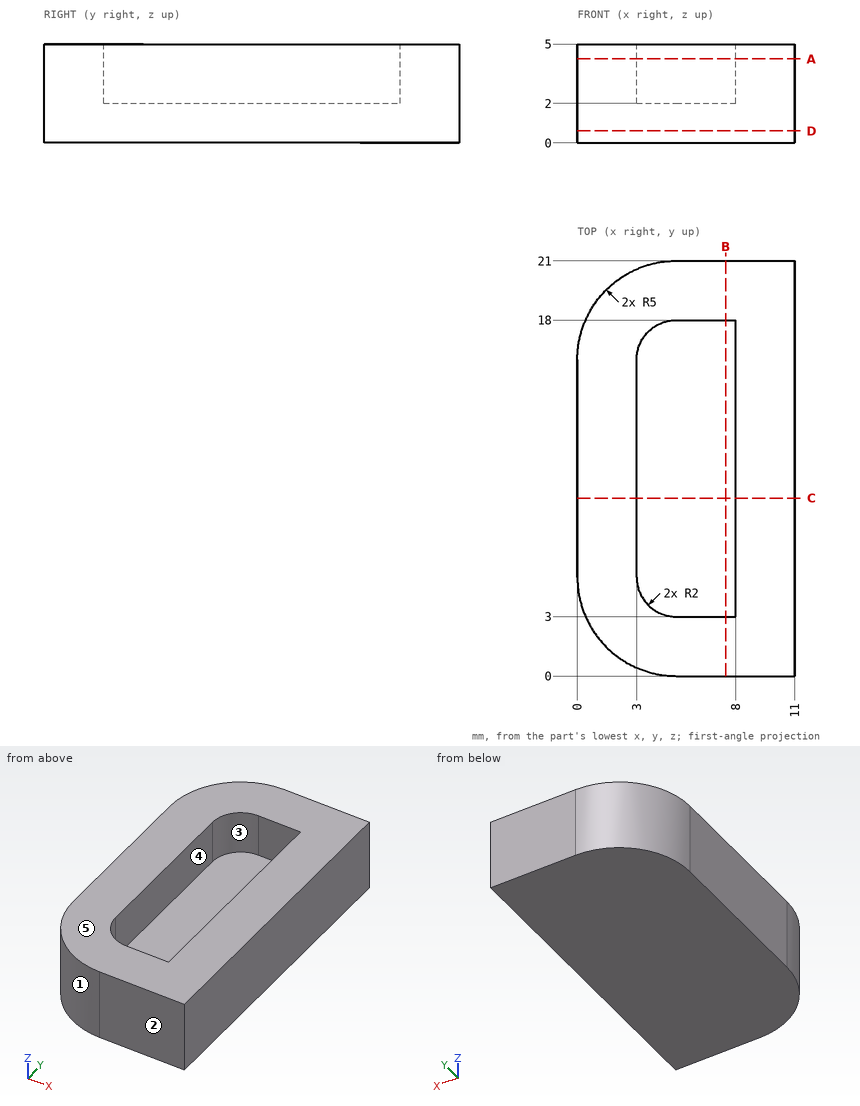
The figure shows three views and two pictorial views of one solid part (mm, origin at its lowest corner). Answer the questions. A direction names the side the tool comes from. Give positions to 0.01 mm unless a question says otherwise; leave off trailing zeros. Loops run counter-clockwise (first coordinate to the right, second up) from the corner with the lowest first, then second, coordinate; pieces in that order, holes last. Notation, with made-up numbers: M -6.5,88 L 43.5,88 A30 ccw 43.5,119 Z; hole C 77.5,62 d3. An arc over 180 degrees is marked long. Write each question's results on one line, items separated by ' | '.
1. A tool of negligible diameter and unlimited length cuts with its end or side. For the marked faces 4 and 5, from which of +Z, -Z, +X, -X, +Y, -Y can it reach the whole face along a straight path? Write none if from no direction.
Values:
face 4: +Z | face 5: +Z, +X, -X, +Y, -Y
2. Section D-D on z = 0.6 is taken. Give the vertices of the cut face in (x, y), plus the area to 3 significant figures.
Values:
outline: M 0,5 A5 ccw 5,0 L 11,0 L 11,21 L 5,21 A5 ccw 0,16 Z | area: 220 mm^2
3. Section C-C on y = 9 is taken. Give the vertices of the cut face in (x, z), plus the area to 3 significant figures.
Values:
outline: M 0,0 L 11,0 L 11,5 L 8,5 L 8,2 L 3,2 L 3,5 L 0,5 Z | area: 40.0 mm^2
4. Section B-B on x = 7.5 is taken. Give the vertices of the cut face in (y, z), plus the area to 3 significant figures.
Values:
outline: M 0,0 L 21,0 L 21,5 L 18,5 L 18,2 L 3,2 L 3,5 L 0,5 Z | area: 60.0 mm^2
5. The mould has two halves that part along X. Classify the marked faces 1, 2 and 3: pulls with the +X half, pulls with the -X half, needs draft (parallel to the pull), parting line crosses it, or undercut.
Values:
face 1: pulls with the -X half | face 2: needs draft | face 3: undercut
6. Section A-A on z = 4.25 is taken. Give the vertices of the cut face in (x, y), plus the area to 3 significant figures.
Values:
outline: M 0,5 A5 ccw 5,0 L 11,0 L 11,21 L 5,21 A5 ccw 0,16 Z; hole M 3,5 A2 ccw 5,3 L 8,3 L 8,18 L 5,18 A2 ccw 3,16 Z | area: 147 mm^2
7. Straight lines are drawn through the part: line 1 (Y direction, x = 6.75, z = 4.4); line 2 (X direction, y = 10.75, z = 3); line 3 (Z direction, x = 4, y = 12.5). For each, find the intervals that lie inside material, in ascending order. Write a range as [from, to].
Values:
line 1: y = [0, 3], [18, 21] | line 2: x = [0, 3], [8, 11] | line 3: z = [0, 2]
8. Given pin 1 (3 mm diameter, centred on x = 2, z = 2.5, fed in from +Y); pin 2 (1 mm diameter, centred on x = 5.5, y = 13.5, fed in from +Z), each flat-ended and moving along its own axis, determine where each tip first touches the part or whether it passes through.
Values:
pin 1: stops at y = 20.77 | pin 2: stops at z = 2
